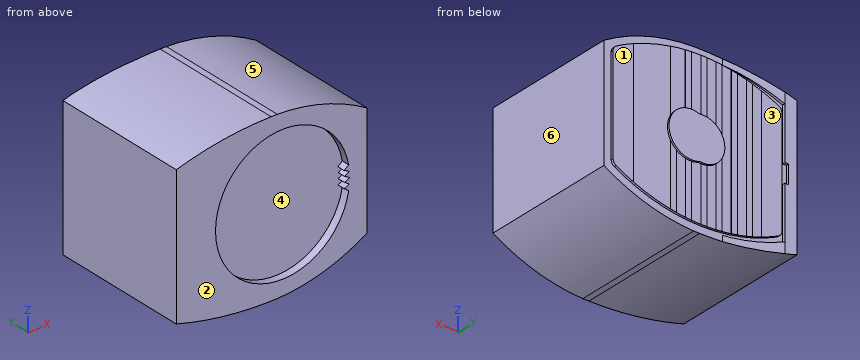
```python
from build123d import *

# Parameters (mm, degrees)
BOSS_EXTRUDE1_DEPTH      = 40
CUT_EXTRUDE1_DEPTH       = 40
CUT_EXTRUDE1_DEPTH_BACK  = 40
CUT_EXTRUDE2_DEPTH       = 40
BOSS_EXTRUDE2_DEPTH      = 0.6223
CUT_EXTRUDE3_DEPTH       = 0.0254
CUT_EXTRUDE4_DEPTH       = 2.032
BOSS_EXTRUDE3_DEPTH      = 0.464
BOSS_EXTRUDE3_DEPTH_BACK = 0.464


with BuildPart() as part:
    # Sketch1 → Boss-Extrude1 (new body)
    with BuildSketch(Plane(origin=(0, -30.021892368, 0), x_dir=(-1, 0, 0), z_dir=(0, -1, 0))):
        with BuildLine():
            Line((-83.1596, 21.651358884), (-84.762120236, 21.651358884))
            ThreePointArc((-84.762120236, 21.651358884), (-96.885117924, 19.694671586), (-108.1278, 14.755258884))
            Line((-108.1278, 14.755258884), (-108.1278, -14.378541116))
            ThreePointArc((-108.1278, -14.378541116), (-96.885117924, -19.317953818), (-84.762120236, -21.274641116))
            Line((-84.762120236, -21.274641116), (-83.1596, -21.274641116))
            ThreePointArc((-83.1596, -21.274641116), (-70.690971885, -20.397039146), (-58.4708, -17.769441116))
            Line((-58.4708, -17.769441116), (-58.4708, 18.146158884))
            ThreePointArc((-58.4708, 18.146158884), (-70.690971885, 20.773756915), (-83.1596, 21.651358884))
        make_face()
    extrude(amount=-BOSS_EXTRUDE1_DEPTH)

    # Sketch2 → Cut-Extrude1 (cut, two sides)
    with BuildSketch(Plane.XY) as cut_extrude1_sk:
        Polygon((54.820843696, 15.118469848), (54.820843696, 6.401707632), (61.6458, 6.401707632), (77.2668, 5.639707632), (110.448229866, 5.639707632), (110.448229866, 15.118469848), align=None)
    extrude(amount=CUT_EXTRUDE1_DEPTH, mode=Mode.SUBTRACT)
    extrude(cut_extrude1_sk.sketch, amount=-CUT_EXTRUDE1_DEPTH_BACK, mode=Mode.SUBTRACT)

    # Sketch3 → Cut-Extrude2 (cut)
    with BuildSketch(Plane(origin=(0, 5.639707632, 0), x_dir=(1, 0, 0), z_dir=(0, 1, 0))):
        with BuildLine():
            Line((60.6298, -2.224641116), (61.6458, -2.224641116))
            Line((61.6458, -2.224641116), (61.6458, -15.889841116))
            ThreePointArc((61.6458, -15.889841116), (69.299882493, -18.411140892), (77.2668, -19.623641116))
            Line((77.2668, -19.623641116), (77.2668, -24.484863345))
            Line((77.2668, -24.484863345), (116.145527093, -24.484863345))
            Line((116.145527093, -24.484863345), (116.145527093, 24.141945465))
            Line((116.145527093, 24.141945465), (77.2668, 24.141945465))
            Line((77.2668, 24.141945465), (77.2668, 20.000358884))
            ThreePointArc((77.2668, 20.000358884), (69.299882493, 18.78785866), (61.6458, 16.266558884))
            Line((61.6458, 16.266558884), (61.6458, 2.601358884))
            Line((61.6458, 2.601358884), (60.6298, 2.601358884))
            Line((60.6298, 2.601358884), (60.6298, -2.224641116))
        make_face()
    extrude(amount=CUT_EXTRUDE2_DEPTH, mode=Mode.SUBTRACT)

    # Sketch4 → Boss-Extrude2 (add)
    with BuildSketch(Plane(origin=(0, 5.639707632, 0), x_dir=(1, 0, 0), z_dir=(0, 1, 0))):
        with BuildLine():
            Line((62.2808, 13.97160372), (62.2808, -13.595028424))
            ThreePointArc((62.2808, -13.595028424), (62.515232291, -14.407180579), (63.146405148, -14.969470936))
            ThreePointArc((63.146405148, -14.969470936), (84.443626018, -19.477271857), (105.437261458, -13.718873038))
            ThreePointArc((105.437261458, -13.718873038), (106.011810141, -13.159417141), (106.2228, -12.385737382))
            Line((106.2228, -12.385737382), (106.2228, 12.76231749))
            ThreePointArc((106.2228, 12.76231749), (106.011758355, 13.536085129), (105.437082995, 14.095551986))
            ThreePointArc((105.437082995, 14.095551986), (84.443582525, 19.852401671), (63.146588971, 15.346134273))
            ThreePointArc((63.146588971, 15.346134273), (62.515286602, 14.783842106), (62.2808, 13.97160372))
        make_face()
    extrude(amount=BOSS_EXTRUDE2_DEPTH)

    # Sketch5 → Cut-Extrude3 (cut)
    with BuildSketch(Plane(origin=(0, 6.236607632, 0), x_dir=(1, 0, 0), z_dir=(0, 1, 0))):
        Polygon((60.8798, -1.974641116), (61.8958, -1.974641116), (61.8958, -15.724128062), (70.725222183, -18.261597014), (77.5168, -19.389388124), (77.5168, -26.279232644), (112.598613265, -26.279232644), (112.598613265, 26.642797699), (77.5168, 26.642797699), (77.5168, 19.766105893), (68.79799987, 18.208824767), (61.8958, 16.100845831), (61.8958, 2.351358884), (60.8798, 2.351358884), align=None)
        with BuildLine():
            Line((106.2228, -12.385737382), (106.2228, 12.76231749))
            ThreePointArc((106.2228, 12.76231749), (106.011758355, 13.536085129), (105.437082995, 14.095551986))
            ThreePointArc((105.437082995, 14.095551986), (103.230284294, 15.241015763), (100.965, 16.26597178))
            Line((100.965, 16.26597178), (100.965, -15.890015871))
            ThreePointArc((100.965, -15.890015871), (103.230393421, -14.864721653), (105.437261458, -13.718873038))
            ThreePointArc((105.437261458, -13.718873038), (106.011810141, -13.159417141), (106.2228, -12.385737382))
        make_face(mode=Mode.SUBTRACT)
        with BuildLine():
            Line((87.4776, -5.556736292), (87.4776, -19.287368321))
            ThreePointArc((87.4776, -19.287368321), (89.400866501, -19.062397708), (91.313, -18.756928734))
            Line((91.313, -18.756928734), (91.313, 19.132183186))
            ThreePointArc((91.313, 19.132183186), (90.526712944, 19.267736149), (89.7382, 19.389675799))
            Line((89.7382, 19.389675799), (89.7382, 4.870687927))
            Line((89.7382, 4.870687927), (87.4776, -5.556736292))
        make_face(mode=Mode.SUBTRACT)
        with BuildLine():
            Line((87.3506, -19.299351408), (87.3506, 19.674500659))
            ThreePointArc((87.3506, 19.674500659), (86.56371005, 19.740853373), (85.7758, 19.79373275))
            Line((85.7758, 19.79373275), (85.7758, -19.418600488))
            ThreePointArc((85.7758, -19.418600488), (86.563710251, -19.365714311), (87.3506, -19.299351408))
        make_face(mode=Mode.SUBTRACT)
        with BuildLine():
            Line((83.3882, -19.496401918), (83.3882, 19.871534346))
            ThreePointArc((83.3882, 19.871534346), (82.60073032, 19.870084861), (81.8134, 19.855199773))
            Line((81.8134, 19.855199773), (81.8134, -19.480050269))
            ThreePointArc((81.8134, -19.480050269), (82.600730229, -19.49494558), (83.3882, -19.496401918))
        make_face(mode=Mode.SUBTRACT)
        with BuildLine():
            Line((79.4258, -19.352519351), (79.4258, 19.727720695))
            ThreePointArc((79.4258, 19.727720695), (78.637747467, 19.658336413), (77.851, 19.575454588))
            Line((77.851, 19.575454588), (77.851, -19.200201536))
            ThreePointArc((77.851, -19.200201536), (78.63774708, -19.283110929), (79.4258, -19.352519351))
        make_face(mode=Mode.SUBTRACT)
        with BuildLine():
            Line((73.8886, 18.948166135), (73.8886, -18.57271762))
            ThreePointArc((73.8886, -18.57271762), (74.674734009, -18.725427281), (75.4634, -18.864469988))
            Line((75.4634, -18.864469988), (75.4634, 19.239829185))
            ThreePointArc((75.4634, 19.239829185), (74.674734726, 19.100829354), (73.8886, 18.948166135))
        make_face(mode=Mode.SUBTRACT)
        with BuildLine():
            Line((69.9262, 17.958552472), (69.9262, -17.58280399))
            ThreePointArc((69.9262, -17.58280399), (70.711659458, -17.808862859), (71.501, -18.020972927))
            Line((71.501, -18.020972927), (71.501, 18.396588518))
            ThreePointArc((71.501, 18.396588518), (70.711660575, 18.184542996), (69.9262, 17.958552472))
        make_face(mode=Mode.SUBTRACT)
        with BuildLine():
            Line((67.5386, -16.801329329), (67.5386, 17.177317791))
            ThreePointArc((67.5386, 17.177317791), (65.318978341, 16.31836829), (63.146588971, 15.346134273))
            ThreePointArc((63.146588971, 15.346134273), (62.515286602, 14.783842106), (62.2808, 13.97160372))
            Line((62.2808, 13.97160372), (62.2808, -13.595028424))
            ThreePointArc((62.2808, -13.595028424), (62.515232309, -14.407180609), (63.146405211, -14.969470967))
            ThreePointArc((63.146405211, -14.969470967), (65.318869691, -15.942064117), (67.5386, -16.801329329))
        make_face(mode=Mode.SUBTRACT)
    extrude(amount=CUT_EXTRUDE3_DEPTH, mode=Mode.SUBTRACT)

    # Sketch6 → Cut-Extrude4 (cut)
    with BuildSketch(Plane(origin=(0, -30.021892368, 0), x_dir=(-1, 0, 0), z_dir=(0, -1, 0))):
        with BuildLine():
            Line((-103.354005387, 3.220690187), (-102.196585301, 2.30003668))
            Line((-102.196585301, 2.30003668), (-103.552849915, 1.710316042))
            Line((-103.552849915, 1.710316042), (-102.319593922, 0.894041707))
            Line((-102.319593922, 0.894041707), (-103.6193, 0.188358884))
            Line((-103.6193, 0.188358884), (-102.319593922, -0.517323938))
            Line((-102.319593922, -0.517323938), (-103.552849915, -1.333598274))
            Line((-103.552849915, -1.333598274), (-102.196585301, -1.923318911))
            Line((-102.196585301, -1.923318911), (-103.354005387, -2.843972418))
            ThreePointArc((-103.354005387, -2.843972418), (-68.6943, 0.188358884), (-103.354005387, 3.220690187))
        make_face()
    extrude(amount=-CUT_EXTRUDE4_DEPTH, mode=Mode.SUBTRACT)

    # Sketch7 → Boss-Extrude3 (add, two sides)
    with BuildSketch(Plane(origin=(0, 6.262007632, 0), x_dir=(1, 0, 0), z_dir=(0, 1, 0))) as boss_extrude3_sk:
        with BuildLine():
            ThreePointArc((84.054570469, -5.319023636), (92.051766601, 0.188358884), (84.054570469, 5.695741404))
            ThreePointArc((84.054570469, 5.695741404), (77.5208, 0.188358884), (84.054570469, -5.319023636))
        make_face()
    extrude(amount=BOSS_EXTRUDE3_DEPTH)
    extrude(boss_extrude3_sk.sketch, amount=-BOSS_EXTRUDE3_DEPTH_BACK)


solid = part.part
```
CAD build for the part. Positions are in the model's coordinates, mm. Face numbers are marked on the shaded views. A direction names the side the tool comes from. Round coordinates to 2 decimals unless told otherwise and drop trailing zeros. Order: outer loops, then holes, each group sorted by start corner. A loop starts at its lowest first (then second) coordinate and runs counter-clockwise, first axis right, second up.
Item 1: Probe line 1 along Z through (x, y) = (82, -7); line 2 along Y through (x, z) = (70.5, 11); line 3 along Y through (x, z) = (87, 2.5). List the from-to ranges inside material, lowest first.
Item 2: Saw through at B-B on x = 66. Write the cut outline in (y, z).
Item 3: Tool access for the marked faces 1, 2 and 3: list every direction of +Z, -Z, +X, -X, +Y, -Y with a clear straight run to the whole face (end or side of a thin tool).
Item 4: Saw through at A-A on y = -16. Write the cut outline in (x, z), then the cut area to 3 significant figures.
Item 5: Mould opens along Z. For the marked faces 4, 5 and 6 say: pulls with the +Z half, pulls with the -Z half, needs draft (parallel to the pull), parting line crosses it, or undercut.
Item 6: Pin check, flat tips, straight feed: pin 1 (1 mm diameter, centred on x = 94.5, y = -5, fed in from -Z); pin 2 (4 mm diameter, centred on x = 104, z = -7.5, fed in from +Y); pin 3 (3 mm diameter, centred on x = 86.5, z = 0.5, fed in from -Y). Stop position of each tip, or through.
Item 7: Saw through at C-C on x = 93. Write the cut outline in (y, z).
Reported:
1. line 1: z = -21.64 to 21.27
1. line 2: y = -30.02 to 6.26
1. line 3: y = -27.99 to 6.73
2. outline: (-30.02, -19.98) - (6.19, -19.98) - (6.19, -17.87) - (5.64, -17.87) - (5.64, -16.6) - (6.26, -16.6) - (6.26, 16.22) - (5.64, 16.22) - (5.64, 17.5) - (6.19, 17.5) - (6.19, 19.6) - (-30.02, 19.6) - close
3. face 1: +Z, -Z, +X, +Y
3. face 2: +Z, -Z, +X, -X, -Y
3. face 3: +Y
4. outline: (58.47, -18.15) arc R88.39 ccw to (83.16, -21.65) - (84.76, -21.65) arc R48.49 ccw to (108.13, -14.76) - (108.13, 14.38) arc R48.49 ccw to (84.76, 21.27) - (83.16, 21.27) arc R88.39 ccw to (58.47, 17.77) - close
4. area: 1,960 mm2
5. face 4: undercut
5. face 5: pulls with the +Z half
5. face 6: needs draft
6. pin 1: stops at z = -20.45
6. pin 2: stops at y = 6.26
6. pin 3: stops at y = -27.99
7. outline: (-30.02, -20.67) - (5.64, -20.67) - (5.64, -18.79) - (6.24, -18.79) - (6.24, 18.42) - (5.64, 18.42) - (5.64, 20.29) - (-30.02, 20.29) - (-30.02, 15.88) - (-27.99, 15.88) - (-27.99, -16.25) - (-30.02, -16.25) - close
